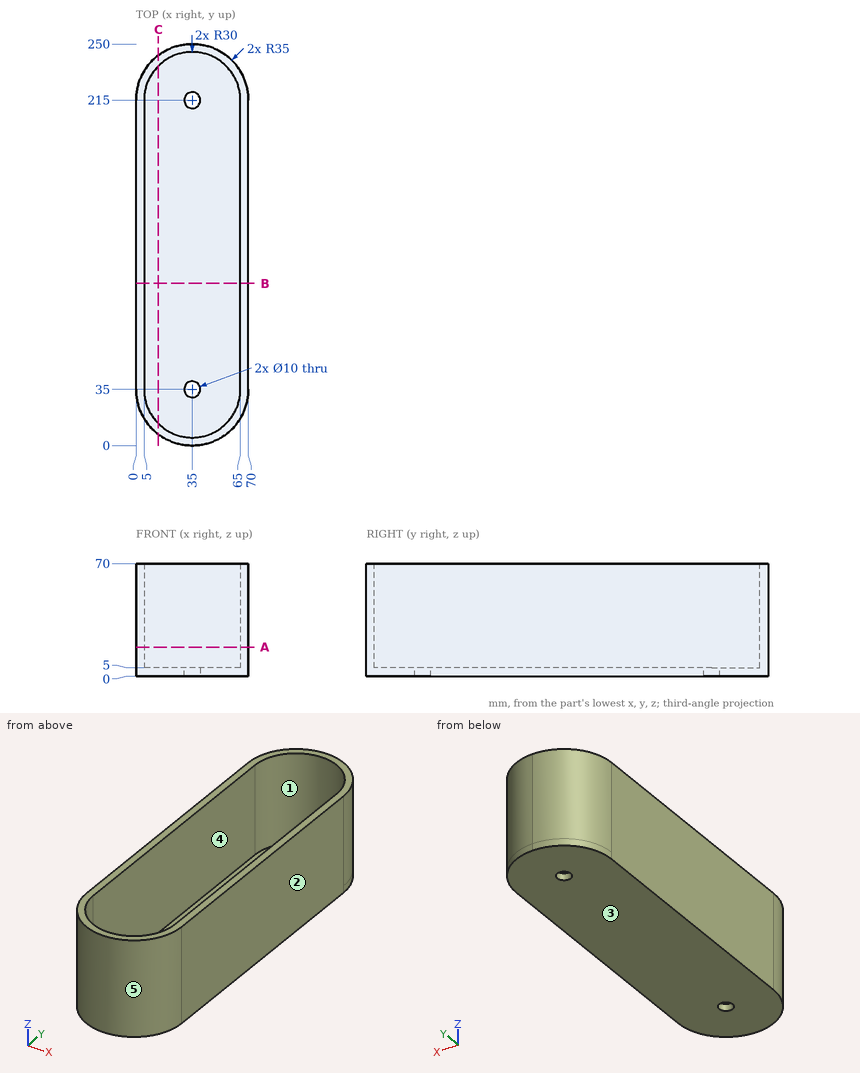
Source: three-view drawing plus pictorial views. Frame: mm from the lowest corner of the part. A direction names the side the tool comes from. Give positions to 0.01 mm unless a question says otherwise; leave off trailing zeros. Loops run counter-clockwise (first coordinate to the right, second up) from the corner with the lowest first, then second, coordinate; pieces in that order, holes last. Notation, with made-up numbers: M 86.5,63 L 93.5,63 A28 cw 93.5,94 Z; hole C 22.25,-19.5 d4. An arc over 180 degrees is marked long. Use CSV: the item, a comma, the result in double quotes.
(1) Pin query (flat end, axial travel): P1, Ø3, axis at x = 54.5, z = 45.5, coming from the -Y side; P2, Ø1, axis at x = 53, z = 10, coming from the +Y side; P3, Ø5, axis at x = 43, z = 49, coming from the +Y side. Return the tip coordinate at first contact, or that it passes through.
Outcome:
P1,"stops at y = 4.98"
P2,"stops at y = 245.31"
P3,"stops at y = 249.57"
(2) Section C-C, the plane x = 14. Return loops of the section in (y, z).
Outcome:
outline,"M 7,0 L 243,0 L 243,70 L 236.42,70 L 236.42,5 L 13.58,5 L 13.58,70 L 7,70 Z"
(3) Material intervals for L1, parallel to X at y = 182, z = 59; L2, parallel to Z at x = 59, y = 95.5; L3, parallel to X at y = 227.5, z = 43, sorted ascending. Write a range as [from, to].
Outcome:
L1,"x = [0, 5], [65, 70]"
L2,"z = [0, 5]"
L3,"x = [2.31, 7.73], [62.27, 67.69]"
(4) Section B-B, the plane y = 101. Return loops of the section in (x, z).
Outcome:
outline,"M 0,0 L 70,0 L 70,70 L 65,70 L 65,5 L 5,5 L 5,70 L 0,70 Z"
(5) Pull-direction query (X, two-part tool) for the marked faces 3, 4 and 5; classes: pulls with the +X half, pulls with the -X half, needs draft (parallel to the pull), parting line crosses it, or undercut.
Outcome:
face 3,"needs draft"
face 4,"undercut"
face 5,"parting line crosses it"
(6) Set-up query: the marked faces 1 and 2. Return all of +Z, -Z, +X, -X, +Y, -Y with unobstructed straight access to the full face (end or side cutting, diameter ignored); none if empty.
Outcome:
face 1,"+Z"
face 2,"+Z, -Z, +X, +Y, -Y"
(7) Section A-A, the plane z = 18. Return loops of the section in (x, y).
Outcome:
outline,"M 0,35 A35 ccw 70,35 L 70,215 A35 ccw 0,215 Z; hole M 5,35 A30 ccw 65,35 L 65,215 A30 ccw 5,215 Z"
